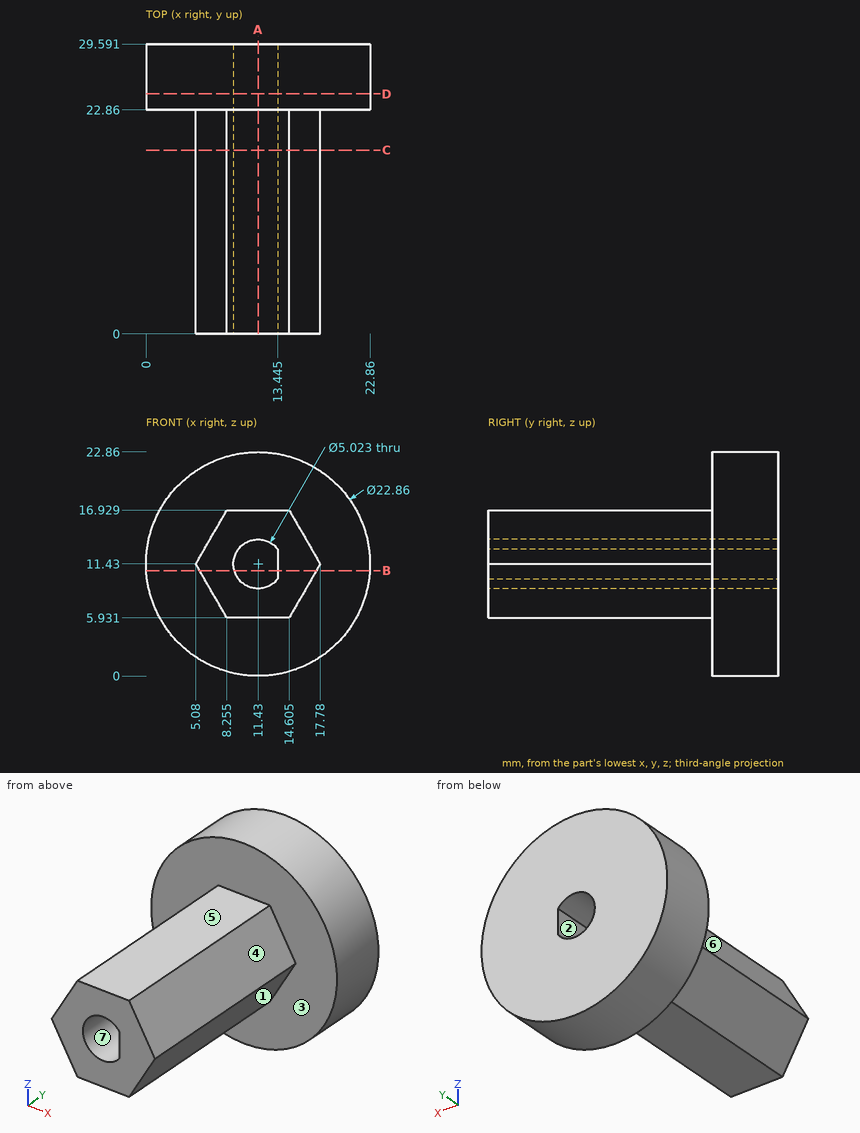
Print and shaded views of the part. All mm, measured from the part's lowest x, y and z. A direction names the side the tool comes from. Coordinates: 2 decimals unless noted, no trailing zeros. Loops run counter-clockwise (first coordinate to the right, second up) from the corner with the lowest first, then second, coordinate; pieces in that order, holes last. Notation, with made-up numbers: M 72.25,-37.75 L 120.25,-37.75 A11 ccw 120.25,-24.75 Z; hole C 78.5,0 d5. An arc over 180 degrees is marked long. Use a Markdown table: item, result. Add a question column.
Q1. Cut at B-B (z = 10.75). Write the cut outline in (x, y) (1 decimal), and give its area (3 significant figures).
Q2. Mould opens along X. For the marked faces 5, 6 and 7 say: +X half, -X half, draft (parallel to the pull), parting line (faces both ways), or undercut.
Q3. Pin check, flat tips, straight feed: P1, Ø12, axis at y = 8.5, z = 9.5, coming from the -X side; P2, Ø12, axis at x = 5.5, y = 19, coming from the -Z side; P3, Ø3, axis at x = 11.5, y = 15, coming from the +Z side. Stop position of each tip, or through.
Q4. Cut at A-A (x = 11.43). Write the cut outline in (y, z).
Q5. Cut at D-D (y = 24.5). Write the cut outline in (x, z) (1 decimal).
Q6. Which spindle directions (+Z, -Z, +X, -X, +Y, -Y) get a long thin tool onto all of the face, cutting with end or side? Do the marked faces 1, 2, 3 and 4. Say none if no direction does.
Q7. Cut at C-C (y = 18.75). Write the cut outline in (x, z) (1 decimal).
Q8. Probe L1, parallel to X at y = 15, z = 11.43 (1 decimal); L2, parallel to Z at x = 11.43, y = 20.5; L3, parallel to Z at x = 11.25, y = 23.5 (1 decimal). List the from-to ranges inside material, lowest first.
Worked out:
| question | item | result |
|---|---|---|
| 1 | outline | M 0,22.9 L 5.5,22.9 L 5.5,0 L 9,0 L 9,29.6 L 0,29.6 Z; M 13.4,0 L 17.4,0 L 17.4,22.9 L 22.8,22.9 L 22.8,29.6 L 13.4,29.6 Z |
| 1 | area | 295 mm2 |
| 2 | face 5 | draft |
| 2 | face 6 | -X half |
| 2 | face 7 | undercut |
| 3 | P1 | stops at x = 5.08 |
| 3 | P2 | stops at z = 0.08 |
| 3 | P3 | stops at z = 16.93 |
| 4 | outline | M 0,5.93 L 22.86,5.93 L 22.86,0 L 29.59,0 L 29.59,8.92 L 0,8.92 Z; M 0,13.94 L 29.59,13.94 L 29.59,22.86 L 22.86,22.86 L 22.86,16.93 L 0,16.93 Z |
| 5 | outline | C 11.4,11.4 d22.9; hole M 13.4,9.9 L 13.4,12.9 A2.5 ccw long Z |
| 6 | face 1 | -Z, +X, -Y |
| 6 | face 2 | +Y, -Y |
| 6 | face 3 | -Y |
| 6 | face 4 | +Z, +X, -Y |
| 7 | outline | M 5.1,11.4 L 8.3,5.9 L 14.6,5.9 L 17.8,11.4 L 14.6,16.9 L 8.3,16.9 Z; hole M 13.4,9.9 L 13.4,12.9 A2.5 ccw long Z |
| 8 | L1 | x = 5.1 to 8.9, 13.4 to 17.8 |
| 8 | L2 | z = 5.93 to 8.92, 13.94 to 16.93 |
| 8 | L3 | z = 0 to 8.9, 13.9 to 22.9 |
